The drawing under review shows one solid part. Ordinate dimensions are in mm from its lowest x, y, z. A direction names the side the tool comes from. Coordinates: 2 decimals unless noted, no trailing zeros. Write each loop counter-clockwise with the first axis right and the second up, starting at its lowest first coordinate (ties: lowest second). Pieces come first, ordered by that corner, then holes.
Q1. Machinability: for the marked faces 1, 2, 3, 4 and 5, which of the approach directions +Z, -Z, +X, -X, +Y, -Y give a long, thin tool a straight path to every point of the face, cutting with its end or side? Answer none if there is none.
Q2. Take a section at B-B (z = 3.5). Give the boundary of the cut face in (x, y).
Q3. Insertion check: pin 1 (1 mm diameter, centred on x = 27.5, z = 36, fed in from -Y); pin 2 (5 mm diameter, centred on y = 88, z = 35, fed in from -X) (3 decimals). Each pin has a flat end and moves straight along its axis. Give the tip position at first contact, or say it passes through.
Q4. Take a section at C-C (x = 30). Give the boundary of the cut face in (y, z) (3 decimals).
Q5. Take a section at D-D (z = 19). Give the boundary of the cut face in (x, y).
Q6. For probe 1 along X at (y, z) = (100, 24); probe 2 along Y at (x, z) = (54.5, 15.5); probe 3 along X at (y, z) = (100, 10), list the stretches that pass through material, from the lowest coordinate up.
Q7. Take a section at A-A (y = 100). Give the boundary of the cut face in (x, z) (3 decimals), and give its area (4 significant figures).
Q8. Mouldability with a two-part tool opening along X and no side actions: class the marked faces 6, 7, 8 and 9 as pulls with the +X half, pulls with the -X half, needs draft (parallel to the pull), parting line crosses it, or undercut.
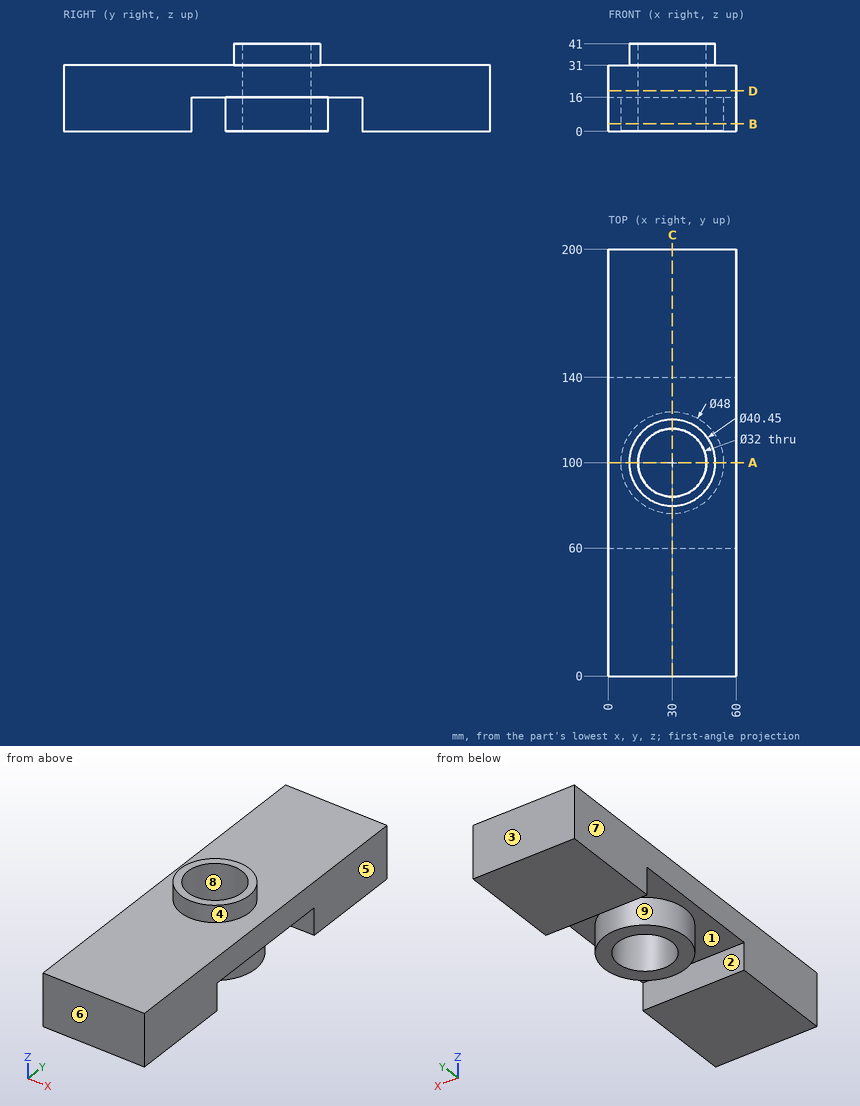
Response:
1. face 1: -Z
1. face 2: -Z, +X, -X
1. face 3: +Z, -Z, +X, -X, +Y
1. face 4: +Z
1. face 5: +Z, -Z, +X, +Y, -Y
2. outline: (0, 0) - (60, 0) - (60, 60) - (0, 60) - close; (0, 140) - (60, 140) - (60, 200) - (0, 200) - close; circle Ø48 at (30, 100); hole circle Ø32 at (30, 100)
3. pin 1: stops at y = 79.87
3. pin 2: stops at x = 12.145
4. outline: (0, 0) - (60, 0) - (60, 16) - (76, 16) - (76, 0) - (84, 0) - (84, 41) - (79.775, 41) - (79.775, 31) - (0, 31) - close; (116, 0) - (124, 0) - (124, 16) - (140, 16) - (140, 0) - (200, 0) - (200, 31) - (120.225, 31) - (120.225, 41) - (116, 41) - close
5. outline: (0, 0) - (60, 0) - (60, 200) - (0, 200) - close; hole circle Ø32 at (30, 100)
6. probe 1: x = 0 to 14, 46 to 60
6. probe 2: y = 0 to 60, 140 to 200
6. probe 3: x = 6 to 14, 46 to 54
7. outline: (0, 16) - (6, 16) - (6, 0) - (14, 0) - (14, 41) - (9.775, 41) - (9.775, 31) - (0, 31) - close; (46, 0) - (54, 0) - (54, 16) - (60, 16) - (60, 31) - (50.225, 31) - (50.225, 41) - (46, 41) - close
7. area: 760.5 mm2
8. face 6: needs draft
8. face 7: pulls with the -X half
8. face 8: undercut
8. face 9: parting line crosses it
